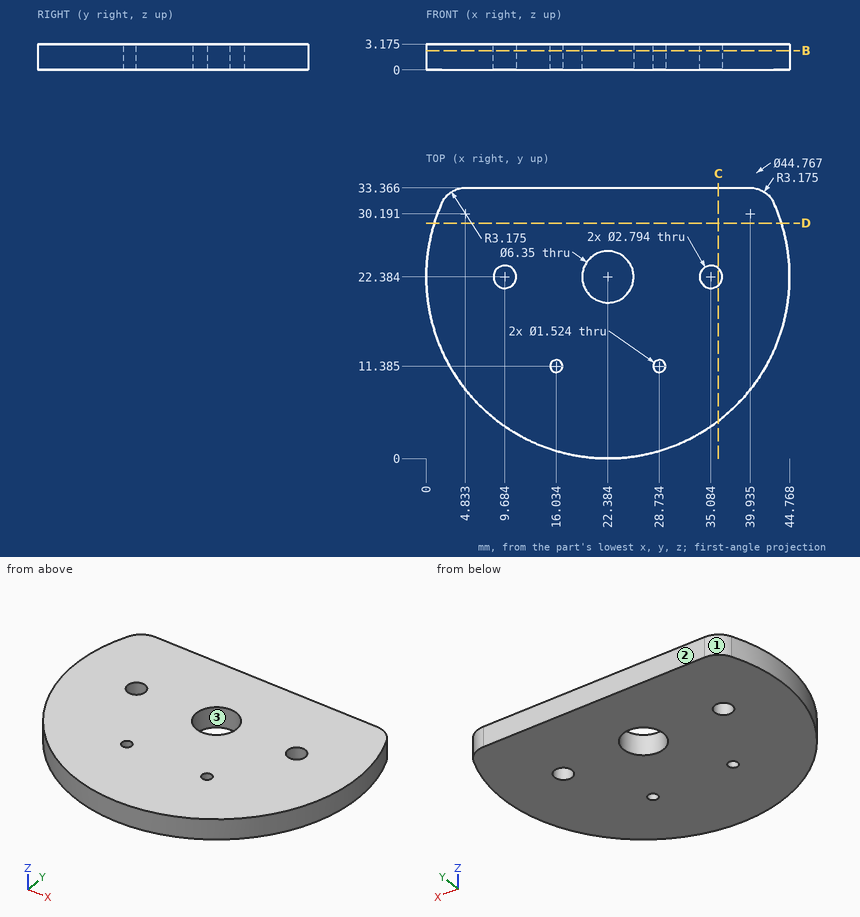
Here's the drawing with two shaded views (mm, measured from the low corner). I have some questions. Round coordinates to 2 decimals unless told otherwise and drop trailing zeros. Loops run counter-clockwise (first coordinate to the right, second up) from the corner with the lowest first, then second, coordinate; pieces in that order, holes last.
1. Thinking about a two-plate mould opening in X: for the marked faces 1, 2 and 3, which applies, released by +X, released by -X, zero draft, split by the parting line, or undercut?
Answers:
face 1: released by -X
face 2: zero draft
face 3: undercut
2. Suppose I cut it at B-B, the plane z = 2.35. Give the number of separate pieces and of enclosed holes in the cut face, and give its area (3 significant figures).
Answers:
separate pieces: 1
enclosed holes: 5
area: 1,210 mm2
3. If I drill on probe 1 along X at (y, z) = (11, 2.2) (1 decimal); probe 2 along X at (y, z) = (8.5, 2) (1 decimal); probe 3 along X at (y, z) = (31, 1.15) (1 decimal), over which ranges is the centre line in solid material (lowest first)?
Answers:
probe 1: x = 3.1 to 15.4, 16.7 to 28.1, 29.4 to 41.7
probe 2: x = 4.8 to 39.9
probe 3: x = 1.7 to 43
4. Suppose I cut it at C-C, the plane x = 36. Please give me the cut outline in (y, z) (1 decimal).
Answers:
outline: (4.6, 0) - (21.3, 0) - (21.3, 3.2) - (4.6, 3.2) - close; (23.4, 0) - (33.4, 0) - (33.4, 3.2) - (23.4, 3.2) - close
5. Will this pin go through, and if not, where does the flat tip stop? pin 1 (1 mm diameter, centred on y = 25.5, z = 2, fed in from +X).
Answers:
pin 1: stops at x = 44.61
6. Suppose I cut it at D-D, the plane y = 29. Please give me the cut outline in (x, z) (1 decimal).
Answers:
outline: (1, 0) - (43.8, 0) - (43.8, 3.2) - (1, 3.2) - close
